Input: part model. Units: mm. Frame: model coordinates. Face numbers are marked on the shaded views. A direction names the side the tool comes from. Give positions to 0.01 mm unless a question says otherwise; leave off trailing zeros. Order: outer loops, then holes, each group sorted by start corner. A loop starts at its lowest first (then second) coordinate and runs counter-clockwise, first axis right, second up. Notation, with made-up numbers: (9.5, 44) - (35.5, 44) arc R10 cw to (35.5, 51) - close; hole circle Ø7 at (23.25, 62). An arc over 180 degrees is marked (long way). Use a Markdown table: item, result.
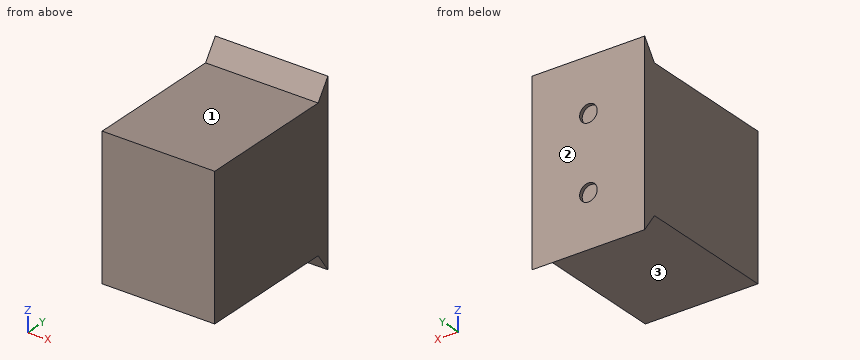
from build123d import *

# Parameters (mm, degrees)
SKETCH1_W           = 4.064
SKETCH1_H           = 5.08
BOSS_EXTRUDE1_DEPTH = 5.08
BOSS_EXTRUDE3_DEPTH = 4.064
SKETCH5_R           = 0.3175
CUT_EXTRUDE2_DEPTH  = 0.127


with BuildPart() as part:
    # Sketch1 → Boss-Extrude1 (new body)
    with BuildSketch(Plane(origin=(0, 0, 0), x_dir=(1, 0, 0), z_dir=(0, 1, 0))):
        Rectangle(SKETCH1_W, SKETCH1_H)
    extrude(amount=BOSS_EXTRUDE1_DEPTH)

    # Sketch4 → Boss-Extrude3 (add)
    with BuildSketch(Plane.ZY.offset(2.032)):
        Polygon((-2.54, 5.08), (-3.220564847, 5.556536636), (3.220564847, 5.556536636), (2.54, 5.08), align=None)
    extrude(amount=-BOSS_EXTRUDE3_DEPTH)

    # Sketch5 → Cut-Extrude2 (cut)
    with BuildSketch(Plane(origin=(0, 5.556536636, 0), x_dir=(1, 0, 0), z_dir=(0, 1, 0))):
        with Locations(Location((0, 1.315564847, 0), (0, 0, 270))):
            Circle(SKETCH5_R)
        with Locations(Location((0, -1.315564847, 0), (0, 0, 90))):
            Circle(SKETCH5_R)
    extrude(amount=-CUT_EXTRUDE2_DEPTH, mode=Mode.SUBTRACT)


solid = part.part
1. Pin query (flat end, axial travel): pin 1 (2 mm diameter, centred on x = -1, y = 4, fed in from -Z). Return the tip coordinate at first contact, or that it passes through.
Response:
| item | result |
|---|---|
| pin 1 | stops at z = -2.54 |
2. Section query C-C (x = 1.55). Return loops of the section in (y, z).
Response:
| item | result |
|---|---|
| outline | (0, -2.54) - (5.08, -2.54) - (5.56, -3.22) - (5.56, 3.22) - (5.08, 2.54) - (0, 2.54) - close |
3. Set-up query: the marked faces 1, 2 and 3. Return all of +Z, -Z, +X, -X, +Y, -Y with unobstructed straight access to the full face (end or side cutting, diameter ignored); none if empty.
Response:
| item | result |
|---|---|
| face 1 | +Z, +X, -X, -Y |
| face 2 | +Z, -Z, +X, -X, +Y |
| face 3 | -Z, +X, -X, -Y |
4. Material intervals for line 1 along Z through (x, y) = (1.1, 0.6); line 2 along Z through (x, y) = (-0.3, 5.2), sorted ascending.
Response:
| item | result |
|---|---|
| line 1 | z = -2.54 to 2.54 |
| line 2 | z = -2.71 to 2.71 |
5. Section query B-B (y = 0.4). Return loops of the section in (x, z).
Response:
| item | result |
|---|---|
| outline | (-2.03, -2.54) - (2.03, -2.54) - (2.03, 2.54) - (-2.03, 2.54) - close |
6. Section query A-A (x = 0). Return loops of the section in (y, z), then the cut area to 3 significant figures.
Response:
| item | result |
|---|---|
| outline | (0, -2.54) - (5.08, -2.54) - (5.56, -3.22) - (5.56, -1.63) - (5.43, -1.63) - (5.43, -1) - (5.56, -1) - (5.56, 1) - (5.43, 1) - (5.43, 1.63) - (5.56, 1.63) - (5.56, 3.22) - (5.08, 2.54) - (0, 2.54) - close |
| area | 28.4 mm^2 |
